```python
from build123d import *

# Parameters (mm, degrees)
SKETCH1_R           = 6.5
SKETCH1_R_2         = 1.5
BOSS_EXTRUDE1_DEPTH = 1.5875
FILLET1_R           = 5
FILLET2_R           = 13


with BuildPart() as part:
    # Sketch1 → Boss-Extrude1 (new body)
    with BuildSketch(Plane.XY):
        Polygon((0, 0), (0, 50), (35, 50), (35, 0), (35, -26), (0, -26), align=None)
        with Locations((17.5, -13)):
            Circle(SKETCH1_R, mode=Mode.SUBTRACT)
        with Locations((5, 45)):
            Circle(SKETCH1_R_2, mode=Mode.SUBTRACT)
        with Locations((5, 25)):
            Circle(SKETCH1_R_2, mode=Mode.SUBTRACT)
        with Locations((5, 5)):
            Circle(SKETCH1_R_2, mode=Mode.SUBTRACT)
        with Locations(Location((30, 5, 0), (0, 0, 180))):
            Circle(SKETCH1_R_2, mode=Mode.SUBTRACT)
        with Locations(Location((30, 25, 0), (0, 0, 180))):
            Circle(SKETCH1_R_2, mode=Mode.SUBTRACT)
        with Locations(Location((30, 45, 0), (0, 0, 180))):
            Circle(SKETCH1_R_2, mode=Mode.SUBTRACT)
    extrude(amount=BOSS_EXTRUDE1_DEPTH)

    # Fillet1
    fillet1_edges = [part.edges().sort_by_distance(p)[0] for p in [
        (0, 50, 0.79375),
        (35, 50, 0.79375),
    ]]
    fillet(fillet1_edges, radius=FILLET1_R)

    # Fillet2
    fillet2_edges = [part.edges().sort_by_distance(p)[0] for p in [
        (35, -26, 0.79375),
        (0, -26, 0.79375),
    ]]
    fillet(fillet2_edges, radius=FILLET2_R)


solid = part.part
```
CAD build for the part. Positions are in the model's coordinates, mm. Give positions to 0.01 mm unless a question says otherwise; leave off trailing zeros. Order: outer loops, then holes, each group sorted by start corner. A loop starts at its lowest first (then second) coordinate and runs counter-clockwise, first axis right, second up.
(1) Saw through at D-D, the plane x = 14. Give the cut face in (y, z).
(2) Saw through at C-C, the plane z = 0.4. Give the cut face in (x, y).
(3) Saw through at A-A, the plane y = 5. Give the cut face in (x, z), then the cut area to 3 significant figures.
(4) Saw through at B-B, the plane x = 17.5. Give the cut face in (y, z), then the cut area to 3 significant figures.
(5) Mould opens along X. For faces 1 (the cylindrical face through (33, 49, 1)), 2 (the cylindrical face through (6.386, 4.425, 0.783)), 3 (the cylindrical face through (31.5, 4.93, 0.78)), 4 (the flat face through (18, 13, 0)) say: released by +X, released by -X, zero draft, split by the parting line, or undercut.
(6) Drill centre lines: L1, parallel to X at y = 46, z = 0.55; L2, parallel to Y at x = 17.5, z = 0.25; L3, parallel to Y at x = 5, z = 0.9. Where is each one in solid material? Low to high.
Results found:
1. outline: (-26, 0) - (-18.48, 0) - (-18.48, 1.59) - (-26, 1.59) - close; (-7.52, 0) - (50, 0) - (50, 1.59) - (-7.52, 1.59) - close
2. outline: (0, -13) arc R13 ccw to (13, -26) - (22, -26) arc R13 ccw to (35, -13) - (35, 45) arc R5 ccw to (30, 50) - (5, 50) arc R5 ccw to (0, 45) - close; hole circle Ø3 at (5, 5); hole circle Ø3 at (5, 25); hole circle Ø3 at (5, 45); hole circle Ø13 at (17.5, -13); hole circle Ø3 at (30, 5); hole circle Ø3 at (30, 25); hole circle Ø3 at (30, 45)
3. outline: (0, 0) - (3.5, 0) - (3.5, 1.59) - (0, 1.59) - close; (6.5, 0) - (28.5, 0) - (28.5, 1.59) - (6.5, 1.59) - close; (31.5, 0) - (35, 0) - (35, 1.59) - (31.5, 1.59) - close
3. area: 46.0 mm2
4. outline: (-26, 0) - (-19.5, 0) - (-19.5, 1.59) - (-26, 1.59) - close; (-6.5, 0) - (50, 0) - (50, 1.59) - (-6.5, 1.59) - close
4. area: 100 mm2
5. face 1: released by +X
5. face 2: undercut
5. face 3: undercut
5. face 4: zero draft
6. L1: x = 0.1 to 3.88, 6.12 to 28.88, 31.12 to 34.9
6. L2: y = -26 to -19.5, -6.5 to 50
6. L3: y = -23.25 to 3.5, 6.5 to 23.5, 26.5 to 43.5, 46.5 to 50
